from build123d import *

# Parameters (mm, degrees)
SKETCH2_W                = 50.8
SKETCH2_H                = 25.4
SKETCH2_W_2              = 44.45
SKETCH2_H_2              = 19.05
EXTRUDE_THIN1_DEPTH      = 457.2
SKETCH25_W               = 50.8
SKETCH25_H               = 25.4
SKETCH25_W_2             = 44.45
SKETCH25_H_2             = 19.05
BOSS_EXTRUDE14_DEPTH     = 25.4
SKETCH29_W               = 50.8
SKETCH29_H               = 25.4
SKETCH29_W_2             = 44.45
SKETCH29_H_2             = 19.05
CUT_EXTRUDE10_DEPTH      = 203.2
SKETCH34_R               = 9.525
SKETCH34_R_2             = 2.15265
CUT_EXTRUDE15_DEPTH      = 25.4
SKETCH35_W               = 50.8
SKETCH35_H               = 25.4
CUT_EXTRUDE16_DEPTH      = 76.2
SKETCH31_R               = 2.15265
CUT_EXTRUDE12_DEPTH      = 1
CUT_EXTRUDE12_DEPTH_BACK = 26.4


with BuildPart() as part:
    # Sketch2 → Extrude-Thin1 (new body)
    with BuildSketch(Plane(origin=(0, 0, 0), x_dir=(1, 0, 0), z_dir=(0, 1, 0))):
        with Locations((10.213756614, 0.671957672)):
            Rectangle(SKETCH2_W, SKETCH2_H)
        with Locations((10.213756614, 0.671957672)):
            Rectangle(SKETCH2_W_2, SKETCH2_H_2, mode=Mode.SUBTRACT)
    extrude(amount=EXTRUDE_THIN1_DEPTH)

    # Sketch25 → Boss-Extrude14 (add)
    with BuildSketch(Plane.XZ):
        with Locations((10.213756614, -0.671957672)):
            Rectangle(SKETCH25_W, SKETCH25_H)
        with Locations((10.213756614, -0.671957672)):
            Rectangle(SKETCH25_W_2, SKETCH25_H_2, mode=Mode.SUBTRACT)
    extrude(amount=BOSS_EXTRUDE14_DEPTH)

    # Sketch29 → Cut-Extrude10 (cut)
    with BuildSketch(Plane(origin=(0, 457.2, 0), x_dir=(1, 0, 0), z_dir=(0, 1, 0))):
        with Locations((10.213756614, 0.671957672)):
            Rectangle(SKETCH29_W, SKETCH29_H)
        with Locations((10.213756614, 0.671957672)):
            Rectangle(SKETCH29_W_2, SKETCH29_H_2, mode=Mode.SUBTRACT)
    extrude(amount=-CUT_EXTRUDE10_DEPTH, mode=Mode.SUBTRACT)

    # Sketch34 → Cut-Extrude15 (cut)
    with BuildSketch(Plane.XY.offset(12.028042328)):
        with Locations((10.213756614, 0)):
            Circle(SKETCH34_R)
        with Locations((29.263756614, 0)):
            Circle(SKETCH34_R_2)
        with Locations((23.684140795, 13.470384182)):
            Circle(SKETCH34_R_2)
        with Locations((10.213756614, 19.05)):
            Circle(SKETCH34_R_2)
        with Locations((-3.256627568, 13.470384182)):
            Circle(SKETCH34_R_2)
        with Locations((-8.836243386, 0)):
            Circle(SKETCH34_R_2)
        with Locations((-3.256627568, -13.470384182)):
            Circle(SKETCH34_R_2)
        with Locations((10.213756614, -19.05)):
            Circle(SKETCH34_R_2)
        with Locations((23.684140795, -13.470384182)):
            Circle(SKETCH34_R_2)
    extrude(amount=-CUT_EXTRUDE15_DEPTH, mode=Mode.SUBTRACT)

    # Sketch35 → Cut-Extrude16 (cut)
    with BuildSketch(Plane(origin=(0, 254, 0), x_dir=(1, 0, 0), z_dir=(0, 1, 0))):
        with Locations((10.213756614, 0.671957672)):
            Rectangle(SKETCH35_W, SKETCH35_H)
    extrude(amount=-CUT_EXTRUDE16_DEPTH, mode=Mode.SUBTRACT)

    # Sketch31 → Cut-Extrude12 (cut, two sides)
    with BuildSketch(Plane(origin=(0, 0, -13.371957672), x_dir=(-1, 0, 0), z_dir=(0, 0, -1))) as cut_extrude12_sk:
        with Locations((-19.738756614, 146.05)):
            Circle(SKETCH31_R)
        with Locations((-0.688756614, 146.05)):
            Circle(SKETCH31_R)
        with Locations((-19.738756614, 171.45)):
            Circle(SKETCH31_R)
        with Locations((-0.688756614, 171.45)):
            Circle(SKETCH31_R)
    extrude(amount=CUT_EXTRUDE12_DEPTH, mode=Mode.SUBTRACT)
    extrude(cut_extrude12_sk.sketch, amount=-CUT_EXTRUDE12_DEPTH_BACK, mode=Mode.SUBTRACT)


solid = part.part
For this review, take the finished solid that the model builds, in its own axes (mm). A direction names the side the tool comes from. Round coordinates to 2 decimals unless told otherwise and drop trailing zeros. Loops run counter-clockwise (first coordinate to the right, second up) from the corner with the lowest first, then second, coordinate; pieces in that order, holes last. Notation, with made-up numbers: (27.5, -12.5) - (70.5, -12.5) arc R16 cw to (70.5, 16.5) - close; hole circle Ø2 at (74.25, -20). An arc over 180 degrees is marked (long way). One line per item, written item: value. Start each with the question number.
Item 1: For faces 5 (the cylindrical face through (-2.3, -15.4, 10.5)), 6 (the flat face through (32.439, 78, -1)), list the 3-axis set-ups (+Z, -Z, +X, -X, +Y, -Y) from which the entire face can be reached by the end or side of a thin tool; tool diameter is ignored.
Item 2: Take a section at D-D (y = 104). Give the boundary of the cut face in (x, z), plus the area to 3 significant figures.
Item 3: For L1, parallel to X at y = 171.45, z = -12.4; L2, parallel to Z at x = 11.5, y = 139.5; L3, parallel to X at y = 138, z = 1, list the stretches that pass through material, from the lowest coordinate up.
Item 4: The part is to be moulded in two halves that separate along Z. For faces 1 (the flat face through (-12.011, 78, -1)), 2 (the cylindrical face through (1.16, 143.95, 10.42)), 3 (the flat face through (10, 78, 8.853)), 4 (the flat face through (10, 78, 12.028)), say which applies: +Z half, -Z half, draft (parallel to the pull), parting line (faces both ways), or undercut.
Item 5: Take a section at C-C (y = 0). State how many separate pieces and enclosed holes the cut face has, plus the area to 3 significant figures.
Item 6: Take a section at A-A (z = -1.5). Give the boundary of the cut face in (x, y), plus the area to 3 significant figures.
Item 7: Take a section at B-B (y = 146.05). Give the boundary of the cut face in (x, z).
Answer below:
1. face 5: +Z, -Z
1. face 6: +Y, -Y
2. outline: (-15.19, -13.37) - (35.61, -13.37) - (35.61, 12.03) - (-15.19, 12.03) - close; hole (-12.01, -10.2) - (32.44, -10.2) - (32.44, 8.85) - (-12.01, 8.85) - close
2. area: 444 mm2
3. L1: x = -15.19 to -1.46, 2.84 to 17.59, 21.89 to 35.61
3. L2: z = -13.37 to -10.2, 8.85 to 12.03
3. L3: x = -15.19 to -12.01, 32.44 to 35.61
4. face 1: undercut
4. face 2: draft
4. face 3: undercut
4. face 4: +Z half
5. separate pieces: 6
5. enclosed holes: 0
5. area: 268 mm2
6. outline: (-15.19, -25.4) - (-12.01, -25.4) - (-12.01, 177.8) - (-15.19, 177.8) - close; (32.44, -25.4) - (35.61, -25.4) - (35.61, 177.8) - (32.44, 177.8) - close
6. area: 1,290 mm2
7. outline: (-15.19, -13.37) - (-1.46, -13.37) - (-1.46, -10.2) - (-12.01, -10.2) - (-12.01, 8.85) - (-1.46, 8.85) - (-1.46, 12.03) - (-15.19, 12.03) - close; (2.84, -13.37) - (17.59, -13.37) - (17.59, -10.2) - (2.84, -10.2) - close; (2.84, 8.85) - (17.59, 8.85) - (17.59, 12.03) - (2.84, 12.03) - close; (21.89, -13.37) - (35.61, -13.37) - (35.61, 12.03) - (21.89, 12.03) - (21.89, 8.85) - (32.44, 8.85) - (32.44, -10.2) - (21.89, -10.2) - close
